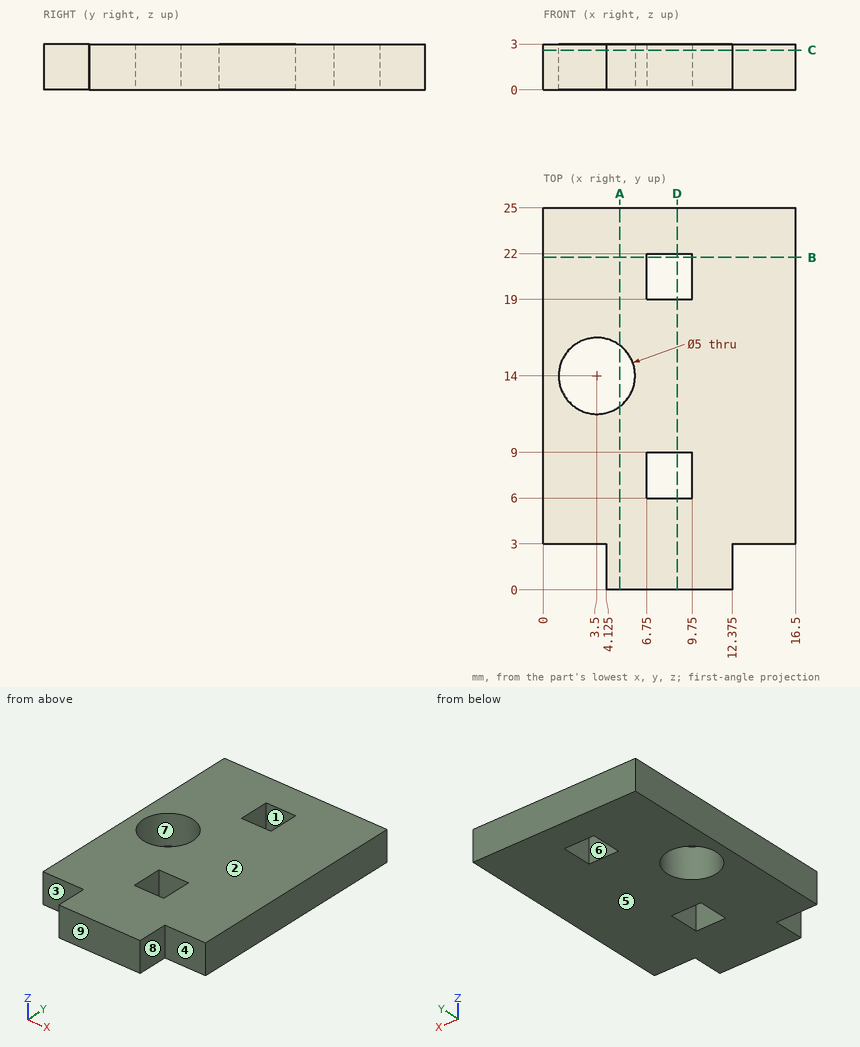
For this review, use the dimensioned drawing (mm, ordinates from the lowest corner) and the shaded views. A direction names the side the tool comes from. Round coordinates to 2 decimals unless told otherwise and drop trailing zeros. Write each loop counter-clockwise with the first axis right and the second up, starting at its lowest first coordinate (ties: lowest second). Pieces come first, ordered by that corner, then holes. Notation, with made-up numbers: (85, 13) -> (109, 13) arc R15 cw to (109, 35) -> close; hole circle Ø11 at (28, 61.5). An arc over 180 degrees is marked (long way). Use CSV: the item, a comma, the result in double quotes.
(1) Consider section A-A, the plane x = 5. Give the boundary of the cut face in (y, z), plus the area to 3 significant figures.
Computed values:
outline,"(0, 0) -> (12, 0) -> (12, 3) -> (0, 3) -> close; (16, 0) -> (25, 0) -> (25, 3) -> (16, 3) -> close"
area,"63.0 mm²"
(2) Consider section C-C, the plane z = 2.6. Give the boundary of the cut face in (x, y) (3 decimals).
Computed values:
outline,"(0, 3) -> (4.125, 3) -> (4.125, 0) -> (12.375, 0) -> (12.375, 3) -> (16.5, 3) -> (16.5, 25) -> (0, 25) -> close; hole circle Ø5 at (3.5, 14); hole (6.75, 6) -> (9.75, 6) -> (9.75, 9) -> (6.75, 9) -> close; hole (6.75, 19) -> (9.75, 19) -> (9.75, 22) -> (6.75, 22) -> close"
(3) Consider section D-D, the plane x = 8.75. Give the boundary of the cut face in (y, z), plus the area to 3 significant figures.
Computed values:
outline,"(0, 0) -> (6, 0) -> (6, 3) -> (0, 3) -> close; (9, 0) -> (19, 0) -> (19, 3) -> (9, 3) -> close; (22, 0) -> (25, 0) -> (25, 3) -> (22, 3) -> close"
area,"57.0 mm²"
(4) Consider section B-B, the plane y = 21.75. Give the boundary of the cut face in (x, z).
Computed values:
outline,"(0, 0) -> (6.75, 0) -> (6.75, 3) -> (0, 3) -> close; (9.75, 0) -> (16.5, 0) -> (16.5, 3) -> (9.75, 3) -> close"
(5) Clearance check with flat-ended pins moving along their axes: P1, Ø0.9, axis at x = 14.5, z = 1, coming from the -Y side; P2, Ø1.5, axis at y = 1.5, z = 2, coming from the -X side (3 decimals). State where each tip first meets the part, or that it passes through.
Computed values:
P1,"y = 3"
P2,"x = 4.125"
(6) Draft analysis for pull direction Y (two halves, no side actions). For the marked faces 6, 7, 8 and 9, state which applies: +Y half, -Y half, draft (parallel to the pull), parting line (faces both ways), or undercut.
Computed values:
face 6,"undercut"
face 7,"undercut"
face 8,"draft"
face 9,"-Y half"
(7) For the marked faces 1, 2, 3, 4 and 5, list the 3-axis set-ups (+Z, -Z, +X, -X, +Y, -Y) from which the entire face can be reached by the end or side of a thin tool; tool diameter is ignored.
Computed values:
face 1,"+Z, -Z"
face 2,"+Z, +X, -X, +Y, -Y"
face 3,"+Z, -Z, -X, -Y"
face 4,"+Z, -Z, +X, -Y"
face 5,"-Z, +X, -X, +Y, -Y"
(8) To check wall thickness, follow L1, parallel to Y at x = 9, z = 0.8; L2, parallel to Y at x = 3.5, z = 1.6; L3, parallel to X at y = 6.5, z = 2.2. State the ranges of each line that lie inside material, in increasing order. Write a range as [from, to].
Computed values:
L1,"[0, 6], [9, 19], [22, 25]"
L2,"[3, 11.5], [16.5, 25]"
L3,"[0, 6.75], [9.75, 16.5]"
